Verification items for the finished model (mm, model axes). Face numbers are marked on the shaded views. Give positions to 0.01 mm unless a question says otherwise; leave off trailing zeros. Order: outer loops, then holes, each group sorted by start corner. A loop starts at its lowest first (then second) coordinate and runs counter-clockwise, first axis right, second up.
from build123d import *

# Parameters (mm, degrees)
F0_W     = 120
F0_H     = 120
F0_R     = 5
F0_R_2   = 21.5
F1_DEPTH = 3.5
F2_DEPTH = 40
F2_TAPER = 2
F3_R     = 5
F4_SIZE2 = 3.49999
F4_SIZE  = 0.49999
F5_R     = 0.5


# Not quite as in the source:
# - a fillet or chamfer is up to 0.001 mm smaller than in the source, because OpenCascade refuses the exact size


with BuildPart() as f1:
    # F0 (on Top) → F1 (new body)
    with BuildSketch(Plane.XY):
        Rectangle(F0_W, F0_H)
        with Locations((-50, -50)):
            Circle(F0_R, mode=Mode.SUBTRACT)
        with Locations((-26, -26)):
            Circle(F0_R_2, mode=Mode.SUBTRACT)
        with Locations((50, -50)):
            Circle(F0_R, mode=Mode.SUBTRACT)
        with Locations((26, -26)):
            Circle(F0_R_2, mode=Mode.SUBTRACT)
        with Locations((-26, 26)):
            Circle(F0_R_2, mode=Mode.SUBTRACT)
        with Locations((-50, 50)):
            Circle(F0_R, mode=Mode.SUBTRACT)
        Circle(F0_R, mode=Mode.SUBTRACT)
        with Locations((26, 26)):
            Circle(F0_R_2, mode=Mode.SUBTRACT)
        with Locations((50, 50)):
            Circle(F0_R, mode=Mode.SUBTRACT)
        with Locations((-50, 50)):
            Circle(F0_R)
        Circle(F0_R)
        with Locations((50, 50)):
            Circle(F0_R)
        with Locations((-50, -50)):
            Circle(F0_R)
        with Locations((50, -50)):
            Circle(F0_R)
    extrude(amount=-F1_DEPTH)

    # F0 (on Top) → F2 (join)
    with BuildSketch(Plane.XY):
        with Locations((-50, 50)):
            Circle(F0_R)
        Circle(F0_R)
        with Locations((50, 50)):
            Circle(F0_R)
        with Locations((50, -50)):
            Circle(F0_R)
        with Locations((-50, -50)):
            Circle(F0_R)
    extrude(amount=F2_DEPTH, taper=F2_TAPER)

    # F3
    f3_edges = [f1.edges().sort_by_distance(p)[0] for p in [
        (-60, -60, -1.75),
        (-60, 60, -1.75),
        (60, 60, -1.75),
        (60, -60, -1.75),
    ]]
    fillet(f3_edges, radius=F3_R)

    # F4 (size 0.5 and 3.5 in the source; OpenCascade refuses exactly that, so slightly less here)
    f4_edges = [f1.edges().sort_by_distance(p)[0] for p in [
        (4.5, 26, -3.5),
        (-47.5, 26, -3.5),
        (-47.5, -26, -3.5),
        (4.5, -26, -3.5),
    ]]
    f4_side = f1.faces().sort_by_distance((0, 0, -3.5))[0]
    chamfer(f4_edges, length=F4_SIZE, length2=F4_SIZE2, reference=f4_side)

    # F5
    f5_edges = [f1.edges().sort_by_distance(p)[0] for p in [
        (0, -60, -3.5),
        (0, -60, 0),
    ]]
    fillet(f5_edges, radius=F5_R)


solid = f1.part
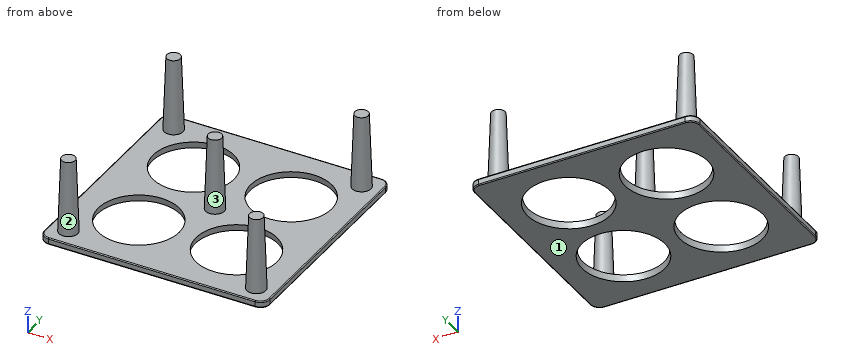
(1) Section check D-D, the plane y = 0. Enter the section's corners in (x, z), then the cut area to 3 significant figures.
Solved:
outline: (-60, -3) arc R0.5 ccw to (-59.5, -3.5) - (59.5, -3.5) arc R0.5 ccw to (60, -3) - (60, -0.5) arc R0.5 ccw to (59.5, 0) - (5, 0) - (3.6, 40) - (-3.6, 40) - (-5, 0) - (-59.5, 0) arc R0.5 ccw to (-60, -0.5) - close
area: 764 mm2
(2) Section check A-A, the plane x = 26. Give the number of separate pieces and of enclosed holes in the cut face, then the cut area to 3 significant figures.
Solved:
separate pieces: 3
enclosed holes: 0
area: 115 mm2
(3) Section check C-C, the plane z = 16. Enter the section's corners in (x, y), then the cut area to 3 significant figures.
Solved:
outline: circle Ø8.88 at (-50, -50); circle Ø8.88 at (-50, 50); circle Ø8.88 at (0, 0); circle Ø8.88 at (50, -50); circle Ø8.88 at (50, 50)
area: 310 mm2
(4) Release check for a two-part mould opening along Y. For the marked faces 1, 2 and 3 record: pulls with the +Y half, pulls with the -Y half, needs draft (parallel to the pull), parting line crosses it, or undercut.
Solved:
face 1: needs draft
face 2: undercut
face 3: parting line crosses it
(5) Go/stop test with flat-tipped pins: pin 1 (12 mm diameter, centred on y = -11.5, z = 26, fed in from +X); pin 2 (3 mm diameter, centred on x = -3, z = 14.5, fed in from +Y); pin 3 (1 mm diameter, centred on x = -1, z = 8, fed in from +Y). Record where each tip stops, or that it passes through.
Solved:
pin 1: passes through
pin 2: stops at y = 4.24
pin 3: stops at y = 4.7
(6) Scan lines: line 1 (Z direction, x = 0.5, y = -49.5); line 2 (Y direction, x = -53, z = 7.5). Record each from-to range of solid material in increasing order.
Solved:
line 1: z = -3.5 to 0
line 2: y = -53.67 to -46.33, 46.33 to 53.67
